Input: dimensioned drawing with shaded views. Units: mm. Origin: part minimum x, y, z. Round coordinates to 2 decimals unless told otherwise and drop trailing zeros. Loops run counter-clockwise (first coordinate to the right, second up) from the corner with the lowest first, then second, coordinate; pieces in that order, holes last. Notation, with made-up numbers: (14, 0) - (44, 0) arc R17 ccw to (44, 10) - close; hole circle Ø8 at (3.25, 6). An arc over 180 degrees is marked (long way). One line per question, with ' | ' between items. Start each with the question number.
1. Pin query (flat end, axial travel): pin 1 (12 mm diameter, centred on y = 393, z = 19, fed in from +X); pin 2 (8 mm diameter, centred on x = 44, y = 693.5, fed in from +Z); pin 3 (6 mm diameter, centred on y = 766.5, z = 40, fed in from +X). Return the tip coordinate at first contact, or that it passes through.
2. Cut plane A-A (y = 692). Return loops of the section in (x, z).
3. Ray query, line 1 (Z direction, x = 7.5, y = 409); line 2 (Z direction, x = 6.5, y = 511.5) (3 decimals); line 3 (X direction, y = 658, z = 41.5). Return the intervals inside material, ascending.
4. Cut plane B-B (z = 16.5). Return loops of the section in (x, y), then the cut area to 3 significant figures.
5. Cut plane C-C (x = 17.5). Return loops of the section in (y, z), then the cut area to 3 significant figures.
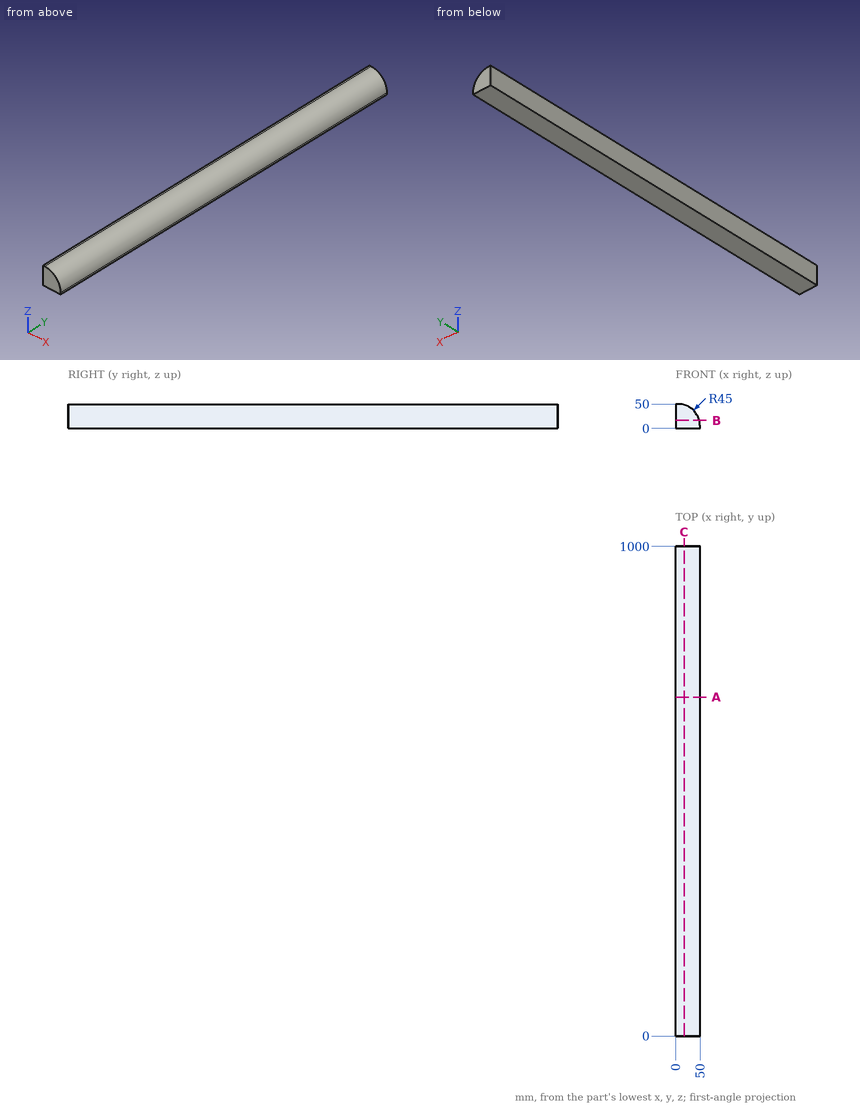
Answers follow:
1) pin 1: stops at x = 49.28 | pin 2: stops at z = 33.28 | pin 3: stops at x = 36.64
2) outline: (0, 0) - (50, 0) - (50, 5) arc R45 ccw to (5, 50) - (0, 50) - close
3) line 1: z = 0 to 49.93 | line 2: z = 0 to 49.975 | line 3: x = 0 to 31.32
4) outline: (0, 0) - (48.51, 0) - (48.51, 1000) - (0, 1000) - close | area: 48,500 mm2
5) outline: (0, 0) - (1000, 0) - (1000, 48.23) - (0, 48.23) - close | area: 48,200 mm2
